The listing builds one solid part. Answer for the finished solid, in the listing's coordinates (mm). A direction names the side the tool comes from. Coordinates: 2 decimals unless noted, no trailing zeros. Write each loop counter-clockwise with the first axis right and the second up, starting at its lowest first coordinate (ties: lowest second). Pieces come first, ordered by that corner, then holes.
(1) Given P1, Ø5, axis at x = 64.5, y = 24.5, coming from the +Z side; P2, Ø2, axis at y = -8.5, z = 8.5, coming from the +X side, each flat-ended and moving along its own axis, determine where each tip first touches the part or whether it passes through.
(2) The part is cut by section C-C on x = 64.5. Determine the outline of the cut face in (y, z).
(3) The part is cut by section A-A on x = -6. Determine the outline of the cut face in (y, z), plus the area to 3 significant figures.
(4) For a pull along Y with two mould halves and no side action, classify faces 1 (the flat face through (-3, -33, 10)), 2 (the flat face through (-32.5, 0, 4)), 3 (the cylindrical face through (72.696, -32.788, -1.268)), 4 (the flat face through (0, 32.5, 4)) as +Y half, -Y half, draft (parallel to the pull), parting line (faces both ways), or undercut.
(5) Straight lines are drawn through the part: line 1 (Y direction, x = 64.5, z = -1.3); line 2 (X direction, y = 18.5, z = 7.75); line 3 (X direction, y = -25, z = -2). For each, find the intervals that lie inside material, in ascending order.
(6) Which of the six approach directions +Z, -Z, +X, -X, +Y, -Y give full straight-line access (tool end or side, diameter ignored) to faces 5 (the flat face through (34.5, 0, 8)), 6 (the cylindrical face through (72.696, 32.788, -1.268)), 7 (the flat face through (0, -32.5, 4))?
(7) The part is cut by section D-D on y = 24.5. Determine the outline of the cut face in (x, z), plus the area to 3 significant figures.
(8) The part is cut by section B-B on y = -3.5. Determine the outline of the cut face in (x, z), plus the area to 3 significant figures.
from build123d import *

# Parameters (mm, degrees)
F0_W         = 69
F0_H         = 69
F0_W_2       = 65
F0_H_2       = 65
F1_DEPTH     = 10
F0_W_3       = 40
F2_DEPTH     = 2.5
F3_R         = 1
F4_T1_DEPTH  = 67
F4_T6_ANGLE  = 359.64
F4_T12_ANGLE = 359.64
F4_T15_DEPTH = 32.5048284938
F5_D         = 4.4


# Not quite as in the source:
# - a fillet or chamfer that OpenCascade refuses, or shapes differently, is made with other operations: its cross-section is extruded or revolved along the edge and cut away or added


with BuildPart() as f1:
    # F0 (on Top) → F1 (new body)
    with BuildSketch(Plane.XY):
        Rectangle(F0_W, F0_H)
        Rectangle(F0_W_2, F0_H_2, mode=Mode.SUBTRACT)
    extrude(amount=F1_DEPTH)

    # F0 (on Top) → F2 (join)
    with BuildSketch(Plane.XY):
        with Locations((54.5, 0)):
            Rectangle(F0_W_3, F0_H)
        Rectangle(F0_W, F0_H)
        Rectangle(F0_W_2, F0_H_2, mode=Mode.SUBTRACT)
    extrude(amount=-F2_DEPTH)

    # F3
    f3_edges = [f1.edges().sort_by_distance(p)[0] for p in [
        (32.5, 32.5, 3.75),
        (-32.5, 32.5, 3.75),
        (-32.5, -32.5, 3.75),
        (32.5, -32.5, 3.75),
        (-34.5, 34.5, 3.75),
        (-34.5, -34.5, 3.75),
        (34.5, 34.5, 5),
        (34.5, -34.5, 5),
    ]]
    fillet(f3_edges, radius=F3_R)

    # F4: fillet of radius 6 on 3 edges, made by hand

    # F4_s2 → F4_t1 (join)
    with BuildSketch(Plane.XZ.offset(-33.5)):
        with BuildLine():
            ThreePointArc((40.5009656854, -0.0004), (36.2573593129, 1.7573593129), (34.4996, 6.0009656854))
            Line((34.4996, 6.0009656854), (33.8994634315, 6.0009656854))
            ThreePointArc((33.8994634315, 6.0009656854), (33.8998634315, 3.0004828427), (33.8998634315, 0))
            Line((33.8998634315, 0), (34.5, -0.6001365685))
            ThreePointArc((34.5, -0.6001365685), (37.5004828427, -0.6001365685), (40.5009656854, -0.6005365685))
            Line((40.5009656854, -0.6005365685), (40.5009656854, -0.0004))
        make_face()
    extrude(amount=F4_T1_DEPTH)


with BuildPart() as f4_tool4:
    # F4_s5 → F4_t6 (revolve)
    with BuildSketch(Plane(origin=(0.2118036776, -33.7091586585, 0), x_dir=(0, 0, 1), z_dir=(0.006283144, -0.9999802609, 0))):
        with BuildLine():
            ThreePointArc((6.0009656854, -34.2884534158), (1.7573593129, -36.0462127287), (-0.0004, -40.2898191013))
            Line((-0.0004, -40.2898191013), (-0.6005365685, -40.2898191013))
            ThreePointArc((-0.6005365685, -40.2898191013), (-0.6001365685, -37.2893362585), (-0.6001365685, -34.2888534158))
            Line((-0.6001365685, -34.2888534158), (0, -33.6887168473))
            ThreePointArc((0, -33.6887168473), (3.0004828427, -33.6887168473), (6.0009656854, -33.6883168473))
            Line((6.0009656854, -33.6883168473), (6.0009656854, -34.2884534158))
        make_face()
    revolve(axis=Axis((33.5, -33.5, 0), (0, 0, 1)), revolution_arc=F4_T6_ANGLE)

    split(bisect_by=Plane.XZ.offset(34.5), keep=Keep.BOTTOM)

    split(bisect_by=Plane.YZ.offset(32.5), keep=Keep.TOP)


with BuildPart() as f1_1:
    add(f1.part)

    # F4_t3: union F4_tool4
    add(f4_tool4.part)


with BuildPart() as f4_tool10:
    # F4_s11 → F4_t12 (revolve)
    with BuildSketch(Plane(origin=(0.2118036776, 33.7091586585, 0), x_dir=(0, 0, 1), z_dir=(0.006283144, 0.9999802609, 0))):
        with BuildLine():
            ThreePointArc((-0.0004, 40.2898191013), (1.7573593129, 36.0462127287), (6.0009656854, 34.2884534158))
            Line((6.0009656854, 34.2884534158), (6.0009656854, 33.6883168473))
            ThreePointArc((6.0009656854, 33.6883168473), (3.0004828427, 33.6887168473), (0, 33.6887168473))
            Line((0, 33.6887168473), (-0.6001365685, 34.2888534158))
            ThreePointArc((-0.6001365685, 34.2888534158), (-0.6001365685, 37.2893362585), (-0.6005365685, 40.2898191013))
            Line((-0.6005365685, 40.2898191013), (-0.0004, 40.2898191013))
        make_face()
    revolve(axis=Axis((33.5, 33.5, 0), (0, 0, -1)), revolution_arc=F4_T12_ANGLE)

    split(bisect_by=Plane.XZ.offset(-34.5), keep=Keep.TOP)

    split(bisect_by=Plane.YZ.offset(32.5), keep=Keep.TOP)


with BuildPart() as f1_2:
    add(f1_1.part)

    # F4_t9: union F4_tool10
    add(f4_tool10.part)

    # F4_s16 → F4_t15 (cut)
    with BuildSketch(Plane.XY.offset(-17.5024142469)):
        with BuildLine():
            ThreePointArc((68.4990343146, 34.5004), (72.7426406871, 32.7426406871), (74.5004, 28.4990343146))
            Line((74.5004, 28.4990343146), (75.1005365685, 28.4990343146))
            ThreePointArc((75.1005365685, 28.4990343146), (75.1001365685, 31.4995171573), (75.1001365685, 34.5))
            Line((75.1001365685, 34.5), (74.5, 35.1001365685))
            ThreePointArc((74.5, 35.1001365685), (71.4995171573, 35.1001365685), (68.4990343146, 35.1005365685))
            Line((68.4990343146, 35.1005365685), (68.4990343146, 34.5004))
        make_face()
        with BuildLine():
            ThreePointArc((68.4990343146, -34.5004), (72.7426406871, -32.7426406871), (74.5004, -28.4990343146))
            Line((74.5004, -28.4990343146), (75.1005365685, -28.4990343146))
            ThreePointArc((75.1005365685, -28.4990343146), (75.1001365685, -31.4995171573), (75.1001365685, -34.5))
            Line((75.1001365685, -34.5), (74.5, -35.1001365685))
            ThreePointArc((74.5, -35.1001365685), (71.4995171573, -35.1001365685), (68.4990343146, -35.1005365685))
            Line((68.4990343146, -35.1005365685), (68.4990343146, -34.5004))
        make_face()
    extrude(amount=F4_T15_DEPTH, mode=Mode.SUBTRACT)

    # F5 (through all)
    with Locations(Plane.XY):
        with Locations((64.5, -24.5), (64.5, 24.5)):
            Hole(F5_D / 2)


solid = f1_2.part
Model answer:
1. P1: stops at z = 0
1. P2: stops at x = 34.5
2. outline: (-34.5, -2.5) - (-26.7, -2.5) - (-26.7, 0) - (-34.5, 0) - close; (-22.3, -2.5) - (22.3, -2.5) - (22.3, 0) - (-22.3, 0) - close; (26.7, -2.5) - (34.5, -2.5) - (34.5, 0) - (26.7, 0) - close
3. outline: (-34.5, -2.5) - (-32.5, -2.5) - (-32.5, 10) - (-34.5, 10) - close; (32.5, -2.5) - (34.5, -2.5) - (34.5, 10) - (32.5, 10) - close
3. area: 50.0 mm2
4. face 1: draft
4. face 2: undercut
4. face 3: -Y half
4. face 4: undercut
5. line 1: y = -34.5 to -26.7, -22.3 to 22.3, 26.7 to 34.5
5. line 2: x = -34.5 to -32.5, 32.5 to 34.5
5. line 3: x = -34.5 to -32.5, 32.5 to 62.36, 66.64 to 74.5
6. face 5: +Z, +X, +Y, -Y
6. face 6: +Z, -Z, +X, +Y
6. face 7: +Z, -Z
7. outline: (-34.5, -2.5) - (-32.5, -2.5) - (-32.5, 10) - (-34.5, 10) - close; (32.5, -2.5) - (62.3, -2.5) - (62.3, 0) - (40.43, 0) arc R6 cw to (34.5, 5.93) - (34.5, 10) - (32.5, 10) - close; (66.7, -2.5) - (74.5, -2.5) - (74.5, 0) - (66.7, 0) - close
7. area: 147 mm2
8. outline: (-34.5, -2.5) - (-32.5, -2.5) - (-32.5, 10) - (-34.5, 10) - close; (32.5, -2.5) - (74.5, -2.5) - (74.5, 0) - (40.43, 0) arc R6 cw to (34.5, 5.93) - (34.5, 10) - (32.5, 10) - close
8. area: 158 mm2
